```python
from build123d import *

# Parameters (mm, degrees)
SKETCH_1_W          = 60
SKETCH_1_H          = 60
EXTRUDE_1_DEPTH     = 4
SKETCH_2_R          = 17.5
CUT_EXTRUDE_1_DEPTH = 44.17406629
HOLE_WIZARD_M3_1_D  = 2.5
HOLE_WIZARD_M5_1_D  = 5.3


with BuildPart() as part:
    # 草圖1 → 填料-伸長1 (new, symmetric)
    with BuildSketch(Plane.XY):
        Rectangle(SKETCH_1_W, SKETCH_1_H)
    extrude(amount=EXTRUDE_1_DEPTH, both=True)

    # 草圖2 → 除料-伸長1 (cut, through all)
    with BuildSketch(Plane.XY.offset(4)):
        Circle(SKETCH_2_R)
    extrude(amount=-CUT_EXTRUDE_1_DEPTH, mode=Mode.SUBTRACT)

    # M3 螺紋孔1 (through all)
    with Locations(Plane.XY.offset(4)):
        with Locations((17.67766953, -17.67766953), (17.67766953, 17.67766953), (-17.67766953, -17.67766953), (-17.67766953, 17.67766953)):
            Hole(HOLE_WIZARD_M3_1_D / 2)

    # M5 餘隙孔1 (through all)
    with Locations(Plane(origin=(0, 30, 0), x_dir=(1, 0, 0), z_dir=(0, 1, 0))):
        with Locations((-25, 0), (25, 0)):
            Hole(HOLE_WIZARD_M5_1_D / 2)


solid = part.part
```
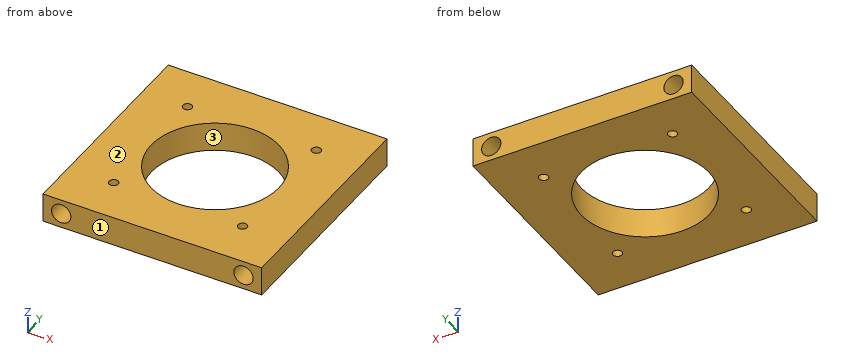
Geometry check sheet. Reference: the model listing, model coordinates, mm. Face numbers are marked on the shaded views. Give positions to 0.01 mm unless a question says otherwise; leave off trailing zeros. Loops run counter-clockwise (first coordinate to the right, second up) from the corner with the lowest first, then second, coordinate; pieces in that order, holes last. Notation, with made-up numbers: (57.25, 88) - (107.25, 88) arc R23 cw to (107.25, 109) - close; hole circle Ø7 at (48, 4). An arc over 180 degrees is marked (long way). Use CSV: the item, a comma, the result in double quotes. Start each with the question number.
Q1. Go/stop test with flat-tipped pins: pin 1 Ø1.5 at (x, y) = (-17.68, -17.68) entering from +Z; pin 2 Ø8 at (x, y) = (-4, 15) entering from +Z. Record where each tip stops, or that it passes through.
Q2. Section check D-D, the plane x = 0. Record the cut outline in (y, z), and give its area (3 significant figures).
Q3. Release check for a two-part mould opening along Y. For the marked faces 1, 2 and 3 record: +Y half, -Y half, draft (parallel to the pull), parting line (faces both ways), or undercut.
Q4. Section check B-B, the plane x = 25. Record the cut outline in (y, z), and give its area (3 significant figures).
Q5. Section check A-A, the plane y = 0. Record the cut outline in (x, z).
Q6. Scan lines: probe 1 along Y at (x, z) = (0, -0.75); probe 2 along X at (y, z) = (-4, 0.75); probe 3 along Y at (x, z) = (6, -3.5). Record each from-to range of solid material in increasing order. Write a range as from..to.
Q7. Section check C-C, the plane z = -1.5. Record the cut outline in (x, y).
Findings below:
1,pin 1,"passes through"
1,pin 2,"stops at z = 4"
2,outline,"(-30, -4) - (-17.5, -4) - (-17.5, 4) - (-30, 4) - close; (17.5, -4) - (30, -4) - (30, 4) - (17.5, 4) - close"
2,area,"200 mm^2"
3,face 1,"-Y half"
3,face 2,"draft"
3,face 3,"undercut"
4,outline,"(-30, -4) - (30, -4) - (30, -2.65) - (-30, -2.65) - close; (-30, 2.65) - (30, 2.65) - (30, 4) - (-30, 4) - close"
4,area,"162 mm^2"
5,outline,"(-30, -4) - (-17.5, -4) - (-17.5, 4) - (-30, 4) - close; (17.5, -4) - (30, -4) - (30, 4) - (17.5, 4) - close; hole circle Ø5.3 at (-25, 0); hole circle Ø5.3 at (25, 0)"
6,probe 1,"y = -30..-17.5, 17.5..30"
6,probe 2,"x = -30..-27.54, -22.46..-17.04, 17.04..22.46, 27.54..30"
6,probe 3,"y = -30..-16.44, 16.44..30"
7,outline,"(-30, -30) - (-27.18, -30) - (-27.18, 30) - (-30, 30) - close; (-22.82, -30) - (22.82, -30) - (22.82, 30) - (-22.82, 30) - close; (27.18, -30) - (30, -30) - (30, 30) - (27.18, 30) - close; hole circle Ø2.5 at (-17.68, -17.68); hole circle Ø2.5 at (-17.68, 17.68); hole circle Ø35 at (0, 0); hole circle Ø2.5 at (17.68, -17.68); hole circle Ø2.5 at (17.68, 17.68)"
